Source: CAD feature listing. Evaluate the final solid. Frame: model axes, mm. Face numbers are marked on the shaded views. A direction names the side the tool comes from. Coordinates: 2 decimals unless noted, no trailing zeros. Loops run counter-clockwise (first coordinate to the right, second up) from the corner with the lowest first, then second, coordinate; pieces in that order, holes last. Notation, with made-up numbers: (74, 78.5) -> (132, 78.5) arc R21 cw to (132, 88.5) -> close; hole circle Ø8 at (87.5, 89). An arc over 180 degrees is marked (long way). One line per question, with ' | ' between items. Start each with the question number.
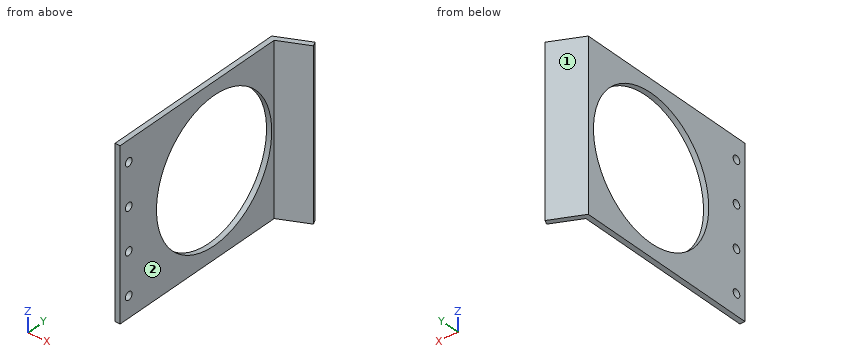
```python
from build123d import *

# Parameters (mm, degrees)
BOSS_EXTRUDE1_DEPTH          = 101.6
F_10_0_1935_DIAMETER_HOLE1_D = 4.9149
SKETCH4_R                    = 42.8625
CUT_EXTRUDE1_DEPTH           = 127


with BuildPart() as part:
    # Sketch1 → Boss-Extrude1 (new body)
    with BuildSketch(Plane.XY):
        Polygon((0, 0), (0, 116.576698078), (19.098350362, 125.48240511), (20.440163343, 122.604877886), (3.175, 114.554), (3.175, 0), align=None)
    extrude(amount=BOSS_EXTRUDE1_DEPTH)

    # #10 (0.1935) Diameter Hole1 (through all)
    with Locations(Plane(origin=(3.175, 0, 0), x_dir=(0, 0, -1), z_dir=(1, 0, 0))):
        with Locations((-88.9, 6.35), (-63.5, 6.35), (-38.1, 6.35), (-12.7, 6.35)):
            Hole(F_10_0_1935_DIAMETER_HOLE1_D / 2)

    # Sketch4 → Cut-Extrude1 (cut)
    with BuildSketch(Plane(origin=(3.175, 0, 0), x_dir=(0, 0, -1), z_dir=(1, 0, 0))):
        with Locations((-50.8, 69.85)):
            Circle(SKETCH4_R)
    extrude(amount=-CUT_EXTRUDE1_DEPTH, mode=Mode.SUBTRACT)


solid = part.part
```
(1) Cut plane C-C, the plane y = 69.85. Return the cut outline in (x, z) (1 decimal).
(2) Cut plane D-D, the plane z = 81. Return the cut outline in (x, y) (3 decimals).
(3) Contact query for flat-ended pins moving along their axis: pin 1 Ø1.5 at (x, z) = (10.5, 59.5) entering from +Y; pin 2 Ø8 at (y, z) = (6.35, 12.7) entering from +X (3 decimals); pin 3 Ø4.5 at (y, z) = (6.35, 88.9) entering from +X; pin 4 Ø12 at (x, z) = (10.5, 52.5) entering from +Y. Output: stop coordinate, or through.
(4) Cut plane A-A, the plane y = 6.35. Return the cut outline in (x, z) (3 decimals), and give its area (3 significant figures).
(5) Ray query, L1, parallel to Y at x = 1.55, z = 12.7; L2, parallel to Y at x = 1.25, z = 63.5; L3, parallel to X at y = 46.5, z = 96.5 (3 decimals). Return the intervals inside material, ascending.
(6) Cut plane B-B, the plane z = 63.5. Return the cut outline in (x, y) (3 decimals), and give its area (3 significant figures).
(7) Access query for the marked faces 1 and 2. Directions: +Z, -Z, +X, -X, +Y, -Y. A direction counts if a zero-diameter tool reaches every point of the face in a straight line with its end or side. Return the directions, or none.
Here are the results:
1) outline: (0, 0) -> (3.2, 0) -> (3.2, 7.9) -> (0, 7.9) -> close; (0, 93.7) -> (3.2, 93.7) -> (3.2, 101.6) -> (0, 101.6) -> close
2) outline: (0, 0) -> (3.175, 0) -> (3.175, 39.434) -> (0, 39.434) -> close; (0, 100.266) -> (3.175, 100.266) -> (3.175, 114.554) -> (20.44, 122.605) -> (19.098, 125.482) -> (0, 116.577) -> close
3) pin 1: stops at y = 121.82 | pin 2: stops at x = 3.175 | pin 3: passes through | pin 4: stops at y = 124.27
4) outline: (0, 0) -> (3.175, 0) -> (3.175, 10.243) -> (0, 10.243) -> close; (0, 15.157) -> (3.175, 15.157) -> (3.175, 35.643) -> (0, 35.643) -> close; (0, 40.557) -> (3.175, 40.557) -> (3.175, 61.043) -> (0, 61.043) -> close; (0, 65.957) -> (3.175, 65.957) -> (3.175, 86.443) -> (0, 86.443) -> close; (0, 91.357) -> (3.175, 91.357) -> (3.175, 101.6) -> (0, 101.6) -> close | area: 260 mm2
5) L1: y = 0 to 3.89, 8.81 to 50.21, 89.49 to 117.3 | L2: y = 0 to 3.89, 8.81 to 28.91, 110.79 to 117.16 | L3: x = 0 to 3.175
6) outline: (0, 0) -> (3.175, 0) -> (3.175, 3.893) -> (0, 3.893) -> close; (0, 8.807) -> (3.175, 8.807) -> (3.175, 28.912) -> (0, 28.912) -> close; (0, 110.788) -> (3.175, 110.788) -> (3.175, 114.554) -> (20.44, 122.605) -> (19.098, 125.482) -> (0, 116.577) -> close | area: 155 mm2
7) face 1: +Z, -Z, -X, +Y | face 2: +Z, -Z, +X, -Y
